Could you check a few things on this model? Use its own coordinates, in mm. A direction names the side the tool comes from. Round coordinates to 2 decimals unless told otherwise and drop trailing zeros. Write each loop counter-clockwise with the first axis right and the second up, starting at its lowest first coordinate (ties: lowest second). Pieces come first, ordered by that corner, then holes. Notation, with made-up numbers: M 0.25,51 L 12.25,51 A21 cw 12.25,88 Z; hole C -26.75,7 d8. An arc over 180 degrees is marked long. One line per item, written item: value. Start each with the question number.
(1) I want a section at D-D on x = -72.5. Please give me the cut outline in (y, z), and give its area (3 significant figures).
(2) I want a section at A-A on x = -102.5. Please give me the cut outline in (y, z), and give its area (3 significant figures).
(3) Which directions (+Z, -Z, +X, -X, +Y, -Y) give clear straight access to the entire face, cutting with the end or side of a thin tool? Please do faces 1 (the face through (-62, -14.082, 10)), 2 (the face through (-140, -0.7, 9.9)), 3 (the face through (-4, 65, 16.582)).
(4) Thinking about a two-plate mould opening in Y: for faces 4 (the face through (-77, 11, 0)), 5 (the face through (-45.754, 7.505, 10.14)), 6 (the face through (-13, 0, 10)), which applies, released by +Y, released by -Y, zero draft, split by the parting line, or undercut?
(5) I'm going to push flat-ended pins straight in: pin 1 Ø6.5 at (y, z) = (-5, 12.5) entering from -X; pin 2 Ø1 at (x, z) = (-86, 16) entering from +Y; pin 3 Ø10 at (x, z) = (-79.5, 8.5) entering from -Y. Where does each tip first touch, or does it pass through?
(6) I want a section at C-C on x = -52.5. Please give me the cut outline in (y, z).
(7) If I drill on L1, parallel to Y at x = -52.5, z = 4.75; L2, parallel to Y at x = -82.5, z = 14; L3, parallel to X at y = 27.5, z = 9.25, over which ranges is the centre line in solid material (lowest first)?
(8) I want a section at B-B on y = 28.5. Please give me the cut outline in (x, z).
```python
from build123d import *

# Parameters (mm, degrees)
SKETCH_1_W                 = 165
SKETCH_1_H                 = 20
EXTRUDE_1_DEPTH            = 15
SKETCH_2_W                 = 7
SKETCH_2_H                 = 20
EXTRUDE_2_DEPTH            = 100
SKETCH_3_R                 = 4.1
CUT_EXTRUDE_1_DEPTH        = 21
PATTERN_LINEAR_1_COUNT     = 8
PATTERN_LINEAR_1_PITCH     = 10
PATTERN_LINEAR_1_COL_COUNT = 8
PATTERN_LINEAR_1_COL_PITCH = 10
CUT_EXTRUDE_2_DEPTH        = 166
SKETCH_5_W                 = 40
SKETCH_5_H                 = 20
EXTRUDE_3_DEPTH            = 15
SKETCH_6_R                 = 4.2
CUT_EXTRUDE_4_DEPTH        = 141
CUT_EXTRUDE_5_DEPTH        = 7
CUT_EXTRUDE_6_DEPTH        = 7
CUT_EXTRUDE_7_DEPTH        = 7
CUT_EXTRUDE_8_DEPTH        = 7
FILLET_1_R                 = 5
FILLET_2_R                 = 5
PATTERN_LINEAR_2_COUNT     = 4
PATTERN_LINEAR_2_PITCH     = 20


with BuildPart() as part:
    # Эскиз1 → Бобышка-Вытянуть1 (new body)
    with BuildSketch(Plane(origin=(0, 0, 0), x_dir=(1, 0, 0), z_dir=(0, 1, 0))):
        with Locations((-82.5, -10)):
            Rectangle(SKETCH_1_W, SKETCH_1_H)
    extrude(amount=EXTRUDE_1_DEPTH)

    # Эскиз2 → Бобышка-Вытянуть2 (add)
    with BuildSketch(Plane(origin=(0, 15, 0), x_dir=(1, 0, 0), z_dir=(0, 1, 0))):
        with Locations((-161.5, -10)):
            Rectangle(SKETCH_2_W, SKETCH_2_H)
        with Locations((-3.5, -10)):
            Rectangle(SKETCH_2_W, SKETCH_2_H)
    extrude(amount=EXTRUDE_2_DEPTH)

    # Эскиз3 → Вырез-Вытянуть1 (cut, through all)
    with BuildSketch(Plane.XY.offset(20)):
        with Locations((-82.5, 10)):
            Circle(SKETCH_3_R)
    cut_extrude_1 = extrude(amount=-CUT_EXTRUDE_1_DEPTH, mode=Mode.SUBTRACT)

    # Линейный массив1: Вырез-Вытянуть1 ×8
    with Locations(*[(-i * PATTERN_LINEAR_1_PITCH, 0, 0) for i in range(1, PATTERN_LINEAR_1_COUNT)]):
        add(cut_extrude_1, mode=Mode.SUBTRACT)

    # Линейный массив1 col: Вырез-Вытянуть1 ×8
    with Locations(*[(i * PATTERN_LINEAR_1_COL_PITCH, 0, 0) for i in range(1, PATTERN_LINEAR_1_COL_COUNT)]):
        add(cut_extrude_1, mode=Mode.SUBTRACT)

    # Эскиз4 → Вырез-Вытянуть2 (cut, through all)
    with BuildSketch(Plane.ZY.offset(165)):
        Polygon((10, 97.4), (16.581793069, 101.2), (16.581793069, 108.8), (10, 112.6), (3.418206931, 108.8), (3.418206931, 101.2), align=None)
    cut_extrude_2 = extrude(amount=-CUT_EXTRUDE_2_DEPTH, mode=Mode.SUBTRACT)

    # Эскиз5 → Бобышка-Вытянуть3 (add)
    with BuildSketch(Plane.XZ):
        with Locations((-120, 10)):
            Rectangle(SKETCH_5_W, SKETCH_5_H)
        with Locations((-45, 10)):
            Rectangle(SKETCH_5_W, SKETCH_5_H)
    extrude(amount=EXTRUDE_3_DEPTH)

    # Эскиз6 → Вырез-Вытянуть4 (cut, through all)
    with BuildSketch(Plane.ZY.offset(140)):
        with Locations((10, -7.5)):
            Circle(SKETCH_6_R)
    extrude(amount=-CUT_EXTRUDE_4_DEPTH, mode=Mode.SUBTRACT)

    # Эскиз7 → Вырез-Вытянуть5 (cut)
    with BuildSketch(Plane.ZY.offset(140)):
        Polygon((17.6, -7.5), (13.8, -0.918206931), (6.2, -0.918206931), (2.4, -7.5), (6.2, -14.081793069), (13.8, -14.081793069), align=None)
    extrude(amount=-CUT_EXTRUDE_5_DEPTH, mode=Mode.SUBTRACT)

    # Эскиз8 → Вырез-Вытянуть6 (cut)
    with BuildSketch(Plane(origin=(-100, 0, 0), x_dir=(0, 0, -1), z_dir=(1, 0, 0))):
        Polygon((-17.6, -7.5), (-13.8, -14.081793069), (-6.2, -14.081793069), (-2.4, -7.5), (-6.2, -0.918206931), (-13.8, -0.918206931), align=None)
    extrude(amount=-CUT_EXTRUDE_6_DEPTH, mode=Mode.SUBTRACT)

    # Эскиз9 → Вырез-Вытянуть7 (cut)
    with BuildSketch(Plane.ZY.offset(65)):
        Polygon((17.6, -7.5), (13.8, -0.918206931), (6.2, -0.918206931), (2.4, -7.5), (6.2, -14.081793069), (13.8, -14.081793069), align=None)
    extrude(amount=-CUT_EXTRUDE_7_DEPTH, mode=Mode.SUBTRACT)

    # Эскиз10 → Вырез-Вытянуть8 (cut)
    with BuildSketch(Plane(origin=(-25, 0, 0), x_dir=(0, 0, -1), z_dir=(1, 0, 0))):
        Polygon((-2.4, -7.5), (-6.2, -0.918206931), (-13.8, -0.918206931), (-17.6, -7.5), (-13.8, -14.081793069), (-6.2, -14.081793069), align=None)
    extrude(amount=-CUT_EXTRUDE_8_DEPTH, mode=Mode.SUBTRACT)

    # Скругление1
    fillet_1_edges = [part.edges().sort_by_distance(p)[0] for p in [
        (-45, -15, 0),
        (-45, -15, 20),
    ]]
    fillet(fillet_1_edges, radius=FILLET_1_R)

    # Скругление2
    fillet_2_edges = [part.edges().sort_by_distance(p)[0] for p in [
        (-120, -15, 0),
        (-120, -15, 20),
    ]]
    fillet(fillet_2_edges, radius=FILLET_2_R)

    # Линейный массив2: Вырез-Вытянуть2 ×4
    with Locations(*[(0, -i * PATTERN_LINEAR_2_PITCH, 0) for i in range(1, PATTERN_LINEAR_2_COUNT)]):
        add(cut_extrude_2, mode=Mode.SUBTRACT)


solid = part.part
```
Found:
1. outline: M 0,0 L 5.9,0 L 5.9,20 L 0,20 Z; M 14.1,0 L 15,0 L 15,20 L 14.1,20 Z
1. area: 136 mm²
2. outline: M -15,5 A5 ccw -10,0 L 5.9,0 L 5.9,20 L -10,20 A5 ccw -15,15 Z; M 14.1,0 L 15,0 L 15,20 L 14.1,20 Z; hole M -14.08,6.2 L -7.5,2.4 L -0.92,6.2 L -0.92,13.8 L -7.5,17.6 L -14.08,13.8 Z
2. area: 275 mm²
3. face 1: none
3. face 2: +Z, -Z, -X, -Y
3. face 3: +X, -X
4. face 4: zero draft
4. face 5: undercut
4. face 6: released by -Y
5. pin 1: stops at x = -140
5. pin 2: stops at y = 15
5. pin 3: stops at y = 0
6. outline: M -15,5 A5 ccw -10,0 L 5.9,0 L 5.9,20 L -10,20 A5 ccw -15,15 Z; M 14.1,0 L 15,0 L 15,20 L 14.1,20 Z; hole C -7.5,10 d8.4
7. L1: y = -14.99 to 5.9, 14.1 to 15
7. L2: y = 0 to 5.9, 14.1 to 15
7. L3: x = -165 to -158, -7 to 0
8. outline: M -165,0 L -158,0 L -158,20 L -165,20 Z; M -7,0 L 0,0 L 0,20 L -7,20 Z
